Input: part model. Units: mm. Frame: model coordinates. Face numbers are marked on the shaded views. Round coordinates to 2 decimals unless told otherwise and drop trailing zeros. Write each loop counter-clockwise with the first axis right and the second up, starting at its lowest first coordinate (ties: lowest second). Pieces come first, ordered by that corner, then holes. Notation, with made-up numbers: (26.5, -19) -> (31.5, -19) arc R16 ccw to (31.5, 5) -> close; hole circle Ø10 at (42.5, 65). An arc over 180 degrees is marked (long way). Use CSV: the item, a comma, the result in double quotes.
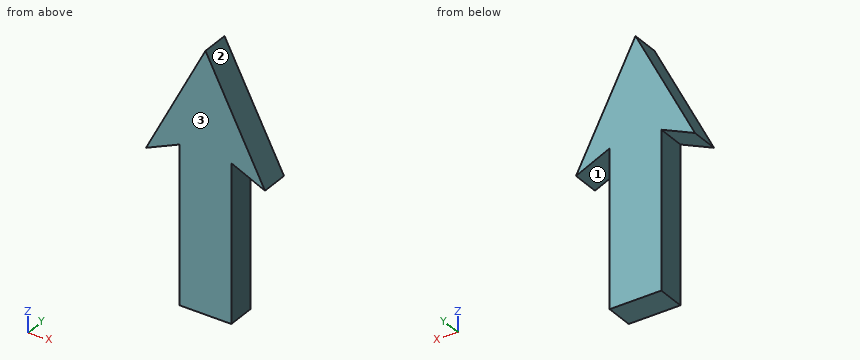
```python
from build123d import *

# Parameters (mm, degrees)
F1_DEPTH = 2.54


with BuildPart() as f1:
    # F0 (on Front) → F1 (new body, symmetric)
    with BuildSketch(Plane.XZ):
        Polygon((0, 46.7954538763), (0, 0), (4.7010933049, 0), (4.7010933049, 28.528785333), (10.8251795173, 25.7835052907), align=None)
    extrude(amount=F1_DEPTH, both=True)

    # F2: F1 across face


with BuildPart() as f1_1:
    add(f1.part)
    add(f1.part.mirror(Plane(origin=(0, 0, 23.3977269381), x_dir=(0, -1, 0), z_dir=(-1, 0, 0))))


solid = f1_1.part
```
Item 1: First-contact query: pin 1 Ø1 at (x, y) = (1.5, -2) entering from +Z; pin 2 Ø1.5 at (y, z) = (1, 20) entering from -X; pin 3 Ø1.5 at (x, y) = (-5.5, -2) entering from -Z. Flat tips, straight axial feed; report the tip coordinate or a pass-through.
Worked answers:
pin 1,"stops at z = 44.85"
pin 2,"stops at x = -4.7"
pin 3,"stops at z = 27.83"
Item 2: Section query D-D on x = -6. Return the cut outline in (y, z).
Worked answers:
outline,"(-2.54, 27.95) -> (2.54, 27.95) -> (2.54, 35.15) -> (-2.54, 35.15) -> close"
Item 3: Section query C-C on z = 15. Return the cut outline in (x, y).
Worked answers:
outline,"(-4.7, -2.54) -> (4.7, -2.54) -> (4.7, 2.54) -> (-4.7, 2.54) -> close"
Item 4: Section query B-B on y = 1.7. Return the cut outline in (x, z), plus the area to 3 significant figures.
Worked answers:
outline,"(-10.83, 25.78) -> (-4.7, 28.53) -> (-4.7, 0) -> (4.7, 0) -> (4.7, 28.53) -> (10.83, 25.78) -> (0, 46.8) -> close"
area,"453 mm²"
Item 5: Pull-direction query (X, two-part tool) for the marked faces 1, 2 and 3; classes: +X half, -X half, draft (parallel to the pull), parting line (faces both ways), or undercut.
Worked answers:
face 1,"undercut"
face 2,"+X half"
face 3,"draft"
Item 6: Line query: line 1 (X direction, y = -0.2, z = 27.5); line 2 (X direction, y = -1.15, z = 27); line 3 (X direction, y = -0.75, z = 12.5). Output: solid intervals per line, ascending.
Worked answers:
line 1,"x = -9.94 to -7, -4.7 to 4.7, 7 to 9.94"
line 2,"x = -10.2 to -8.11, -4.7 to 4.7, 8.11 to 10.2"
line 3,"x = -4.7 to 4.7"
Item 7: Section query A-A on z = 27. Return the cut outline in (x, y), plus the area to 3 significant figures.
Worked answers:
outline,"(-10.2, -2.54) -> (-8.11, -2.54) -> (-8.11, 2.54) -> (-10.2, 2.54) -> close; (-4.7, -2.54) -> (4.7, -2.54) -> (4.7, 2.54) -> (-4.7, 2.54) -> close; (8.11, -2.54) -> (10.2, -2.54) -> (10.2, 2.54) -> (8.11, 2.54) -> close"
area,"69.0 mm²"
